Source: CAD feature listing. Evaluate the final solid. Frame: model axes, mm. A direction names the side the tool comes from. Coordinates: 2 decimals unless noted, no trailing zeros. Write each loop counter-clockwise with the first axis right and the second up, starting at its lowest first coordinate (ties: lowest second). Pieces come first, ordered by that corner, then holes. Notation, with made-up numbers: (33, -5.75) -> (68, -5.75) arc R14 ccw to (68, 10.25) -> close; hole circle Ø5 at (39.5, 47). An arc over 180 degrees is marked (long way). Write item = value, one per line.
Autodesk Inventor part; units mm, degrees
ref_plane "YZ Plane" through (0, 0, 0) normal (1, 0, 0) x (0, 1, 0)
ref_plane "XZ Plane" through (0, 0, 0) normal (0, 1, 0) x (-1, 0, 0)
ref_plane "XY Plane" through (0, 0, 0) normal (0, 0, 1) x (1, 0, 0)
sketch "Sketch1" plane through (0, 0, 0) normal (0, 1, 0) x (-1, 0, 0)
  line L0 (0, 0) -> (38.1, 0)
  line L1 (38.1, 0) -> (38.1, -88.9)
  line L2 (38.1, -88.9) -> (0, -88.9)
  line L3 (0, -88.9) -> (0, 0)
  dimension "d0" = 88.9
  dimension "d1" = 38.1
extrude "Extrusion1" add sketch "Sketch1" along normal blind 58.0644
sketch "Sketch6" plane through (0, 58.0644, 0) normal (0, 1, 0) x (1, 0, 0)
  line L0 (-38.1, 0) -> (0, 0)
  line L1 (0, 0) -> (0, 88.9)
  line L2 (0, 88.9) -> (-38.1, 88.9)
  line L3 (-38.1, 88.9) -> (-38.1, 0)
  line L4 (-38.1, 0) -> (-6.35, 0)
  line L5 (-6.35, 0) -> (-6.35, 88.9)
  line L6 (-6.35, 88.9) -> (-38.1, 88.9)
  line L7 (-38.1, 88.9) -> (-38.1, 0)
  dimension "d38" = 0
  dimension "d39" = 31.75
  dimension "d40" = 0
  dimension "d41" = 88.9
extrude "Extrusion5" cut sketch "Sketch6" against normal blind 12.7 contours L3 L2 L5 L0
sketch "Sketch7" plane through (0, 45.3644, 0) normal (0, 1, 0) x (1, 0, 0)
  arc A0 (-20.2095, 23.7057) -> (-20.2095, 11.2193) centre (-19.05, 17.4625) ccw
  line L0 (-26.5557, 23.7057) -> (-20.2095, 23.7057)
  line L1 (-26.5557, 11.2193) -> (-26.5557, 23.7057)
  line L2 (-26.5557, 11.2193) -> (-20.2095, 11.2193)
  arc A1 (-17.8905, 11.2193) -> (-17.8905, 23.7057) centre (-19.05, 17.4625) ccw
  line L3 (-17.8905, 11.2193) -> (-11.5443, 11.2193)
  line L4 (-11.5443, 23.7057) -> (-11.5443, 11.2193)
  line L5 (-17.8905, 23.7057) -> (-11.5443, 23.7057)
  arc A2 (-25.2932, 70.278) -> (-12.8068, 70.278) centre (-19.05, 71.4375) ccw
  line L6 (-25.2932, 70.278) -> (-25.2932, 63.9318)
  line L7 (-12.8068, 63.9318) -> (-25.2932, 63.9318)
  line L8 (-12.8068, 70.278) -> (-12.8068, 63.9318)
  arc A3 (-12.8068, 72.597) -> (-25.2932, 72.597) centre (-19.05, 71.4375) ccw
  line L9 (-12.8068, 78.9432) -> (-12.8068, 72.597)
  line L10 (-25.2932, 78.9432) -> (-12.8068, 78.9432)
  line L11 (-25.2932, 78.9432) -> (-25.2932, 72.597)
  circle A4 centre (-19.05, 52.3875) radius 1.7526
  circle A5 centre (-19.05, 39.6875) radius 1.7526
  point P0 (0, 0)
hole "Hole2" at (-19.05, 45.3644, -71.4375) at (-19.05, 45.3644, -17.4625) direction (0, -1, 0) diameter 9.525 depth 6.35 tip angle 118
sketch "Sketch8" plane through (0, 45.3644, 0) normal (0, 1, 0) x (1, 0, 0)
  circle A0 centre (-19.05, 52.3875) radius 1.7526
  circle A1 centre (-19.05, 39.6875) radius 1.7526
  point P0 (0, 0)
hole "Hole3" at (-19.05, 45.3644, -52.3875) at (-19.05, 45.3644, -39.6875) direction (0, -1, 0) diameter 3.5052 depth 6.35 tip angle 118
sketch "Sketch9" plane through (0, 0, 0) normal (0, -1, 0) x (1, 0, 0)
  line L0 (0, 0) -> (-38.1, 0)
  line L1 (-38.1, 0) -> (-38.1, -88.9)
  line L2 (-38.1, -88.9) -> (0, -88.9)
  line L3 (0, -88.9) -> (0, 0)
  circle A0 centre (-19.05, -17.4625) radius 4.7625
  circle A1 centre (-19.05, -71.4375) radius 4.7625
  circle A2 centre (-19.05, -39.6875) radius 1.7526
  circle A3 centre (-19.05, -52.3875) radius 1.7526
  circle A4 centre (-19.05, -39.6875) radius 1.7526
  circle A5 centre (-19.05, -52.3875) radius 1.7526
hole "Hole4" at (-19.05, 0, -17.4625) at (-19.05, 0, -71.4375) at (-19.05, 0, -39.6875) at (-19.05, 0, -52.3875) direction (0, 1, 0) diameter 3.5052 depth 6.35 tip angle 118
thread "Thread1"
thread "Thread2"
thread "Thread3"
thread "Thread4"
thread "Thread5"
thread "Thread6"
properties part number "TSV-Support"
1) Material intervals for probe 1 along Z at (x, y) = (-19.05, 1.75); probe 2 along Z at (x, y) = (-19.05, 43.5) (3 decimals); probe 3 along Y at (x, z) = (-33.5, -51), sorted ascending. Write a range as [from, to].
Answer block:
probe_1 = [-88.9, -73.19], [-69.68, -54.14], [-50.63, -41.44], [-37.93, -19.22], [-15.71, 0]
probe_2 = [-88.9, -76.2], [-66.675, -54.14], [-50.635, -41.44], [-37.935, -22.225], [-12.7, 0]
probe_3 = [0, 45.36]
2) First-contact query: pin 1 Ø1.5 at (x, y) = (-4, 15) entering from +Z; pin 2 Ø3 at (x, z) = (-19.05, -52.39) entering from -Y; pin 3 Ø4.5 at (x, z) = (-19.05, -17.46) entering from +Y; pin 4 Ø5.5 at (x, z) = (-19.05, -71.44) entering from +Y. Flat tips, straight axial feed; report the tip coordinate or a pass-through.
Answer block:
pin_1 = 0
pin_2 = 6.5
pin_3 = 37.51
pin_4 = 37.81
3) Reachability of faces 1 (the cylindrical face through (-22.27, 42.14, -20.97)), 2 (the flat face through (-6.35, 52, -44)), 3 (the cylindrical face through (-18.38, 3.22, -19.08)) from +Z, -Z, +X, -X, +Y, -Y: full face, straight path, thin tool, end or side. Return the list, or none.
Answer block:
face_1 = +Y
face_2 = +Z, -Z, -X, +Y
face_3 = -Y
4) Cut plane A-A, the plane z = -10. Output: boundary loops of the cut face in (x, y).
Answer block:
outline = (-38.1, 0) -> (0, 0) -> (0, 58.06) -> (-6.35, 58.06) -> (-6.35, 45.36) -> (-38.1, 45.36) -> close
5) Pull-direction query (X, two-part tool) for faces 4 (the cylindrical face through (-17.98, 3.22, -38.3)), 5 (the flat face through (-22, 45.364, -45)), 6 (the flat face through (0, 29, -45)); classes: +X half, -X half, draft (parallel to the pull), parting line (faces both ways), or undercut.
Answer block:
face_4 = undercut
face_5 = draft
face_6 = +X half
6) Cut plane B-B, the plane y = 53. Output: boundary loops of the cut face in (x, z).
Answer block:
outline = (-6.35, -88.9) -> (0, -88.9) -> (0, 0) -> (-6.35, 0) -> close
